The listing builds one solid part. Answer for the finished solid, in the listing's coordinates (mm). A direction names the side the tool comes from. Coordinates: 2 decimals unless noted, no trailing zeros. Write each loop counter-clockwise with the first axis right and the second up, starting at its lowest first coordinate (ties: lowest second). Pieces come first, ordered by that corner, then holes.
(1) Straight lines are drawn through the part: line 1 (X direction, y = -1, z = 19); line 2 (X direction, y = -9.5, z = 23.5). For each, find the intervals that lie inside material, in ascending order.
(2) The part is cut by section C-C on x = -19.5. Determine the outline of the cut face in (y, z), plus the area to 3 significant figures.
(3) Given P1, Ø4, axis at y = 10.5, z = 5, coming from the -X side; P2, Ø8, axis at x = -5.5, y = -4, coming from the -Z side, each flat-ended and moving along its own axis, determine where each tip first touches the part or whether it passes through.
(4) For a pull along Y with two mould halves and no side action, classify faces 1 (the cylindrical face through (-12.215, -12.199, 12.661)), 2 (the flat face through (-3, 12.5, 12)), 3 (the cylindrical face through (0.105, 8.801, 24.715)) as +Y half, -Y half, draft (parallel to the pull), parting line (faces both ways), or undercut.
(5) The part is cut by section B-B on x = -14.5. Determine the outline of the cut face in (y, z).
(6) The part is cut by section A-A on z = 6.25. Determine the outline of the cut face in (x, y), plus the area to 3 significant figures.
(7) Which of the six approach directions +Z, -Z, +X, -X, +Y, -Y give full straight-line access (tool end or side, diameter ignored) to faces 4 (the cylindrical face through (8.801, -0.105, 0.285)), 5 (the cylindrical face through (-8.215, 8.199, 12.339)), 6 (the cylindrical face through (8.801, -0.105, 24.715))?
from build123d import *

# Parameters (mm, degrees)
SKETCH1_W           = 25
SKETCH1_H           = 25
BOSS_EXTRUDE1_DEPTH = 25
SKETCH3_R           = 2.25
BOSS_EXTRUDE2_DEPTH = 10
BOSS_EXTRUDE2_TAPER = 2
SKETCH4_R           = 2.25
BOSS_EXTRUDE3_DEPTH = 10
BOSS_EXTRUDE3_TAPER = 2
CUT_EXTRUDE1_DEPTH  = 25
FILLET1_R           = 1


with BuildPart() as part:
    # Sketch1 → Boss-Extrude1 (new body)
    with BuildSketch(Plane.XY):
        Rectangle(SKETCH1_W, SKETCH1_H)
    extrude(amount=BOSS_EXTRUDE1_DEPTH)

    # Sketch3 → Boss-Extrude2 (add)
    with BuildSketch(Plane.ZY.offset(12.5)):
        with Locations((12.5, 0)):
            Circle(SKETCH3_R)
    extrude(amount=BOSS_EXTRUDE2_DEPTH, taper=BOSS_EXTRUDE2_TAPER)

    # Sketch4 → Boss-Extrude3 (add)
    with BuildSketch(Plane(origin=(0, 12.5, 0), x_dir=(1, 0, 0), z_dir=(0, 1, 0))):
        with Locations((1e-09, -12.5)):
            Circle(SKETCH4_R)
    extrude(amount=BOSS_EXTRUDE3_DEPTH, taper=BOSS_EXTRUDE3_TAPER)

    # Sketch5 → Cut-Extrude1 (cut)
    with BuildSketch(Plane(origin=(0, 0, 0), x_dir=(-1, 0, 0), z_dir=(0, 0, -1))):
        with BuildLine():
            Line((-7.5, -8.5), (7.5, -8.5))
            ThreePointArc((7.5, -8.5), (8.207106781, -8.207106781), (8.5, -7.5))
            Line((8.5, -7.5), (8.5, 7.5))
            ThreePointArc((8.5, 7.5), (8.207106781, 8.207106781), (7.5, 8.5))
            Line((7.5, 8.5), (-7.5, 8.5))
            ThreePointArc((-7.5, 8.5), (-8.207106781, 8.207106781), (-8.5, 7.5))
            Line((-8.5, 7.5), (-8.5, -7.5))
            ThreePointArc((-8.5, -7.5), (-8.207106781, -8.207106781), (-7.5, -8.5))
        make_face()
    extrude(amount=-CUT_EXTRUDE1_DEPTH, mode=Mode.SUBTRACT)

    # Fillet1
    fillet1_edges = [part.edges().sort_by_distance(p)[0] for p in [
        (-12.5, 0, 25),
        (0, -12.5, 25),
        (-22.5, 0, 10.599207695),
        (-1.900792304, 22.5, 12.5),
        (8.207106781, -8.207106781, 0),
        (0, -8.5, 0),
        (-8.207106781, -8.207106781, 0),
        (-8.5, 0, 0),
        (-8.207106781, 8.207106781, 0),
        (0, 8.5, 0),
        (8.207106781, 8.207106781, 0),
        (8.5, 0, 0),
        (8.207106781, -8.207106781, 25),
        (8.5, 0, 25),
        (8.207106781, 8.207106781, 25),
        (0, 8.5, 25),
        (-8.207106781, 8.207106781, 25),
        (-8.5, 0, 25),
        (-8.207106781, -8.207106781, 25),
        (0, -8.5, 25),
        (12.5, 0, 25),
        (0, -12.5, 0),
        (-12.5, 0, 0),
        (0, 12.5, 0),
        (12.5, 0, 0),
        (0, 12.5, 25),
        (12.5, -12.5, 12.5),
        (-12.5, -12.5, 12.5),
        (-12.5, 12.5, 12.5),
        (12.5, 12.5, 12.5),
    ]]
    fillet(fillet1_edges, radius=FILLET1_R)


solid = part.part
Model answer:
1. line 1: x = -12.5 to -8.5, 8.5 to 12.5
1. line 2: x = -12.5 to 12.5
2. outline: circle Ø4.01 at (0, 12.5)
2. area: 12.6 mm2
3. P1: stops at x = -12.5
3. P2: stops at z = 0
4. face 1: -Y half
4. face 2: +Y half
4. face 3: undercut
5. outline: circle Ø4.36 at (0, 12.5)
6. outline: (-12.5, -11.5) arc R1 ccw to (-11.5, -12.5) - (11.5, -12.5) arc R1 ccw to (12.5, -11.5) - (12.5, 11.5) arc R1 ccw to (11.5, 12.5) - (-11.5, 12.5) arc R1 ccw to (-12.5, 11.5) - close; hole (-8.5, -7.5) arc R1 ccw to (-7.5, -8.5) - (7.5, -8.5) arc R1 ccw to (8.5, -7.5) - (8.5, 7.5) arc R1 ccw to (7.5, 8.5) - (-7.5, 8.5) arc R1 ccw to (-8.5, 7.5) - close
6. area: 336 mm2
7. face 4: -Z
7. face 5: +Z, -Z
7. face 6: +Z
